from build123d import *

# Parameters (mm, degrees)
F1_DEPTH = 400
F2_R     = 2.15
F3_DEPTH = 800
F4_R     = 2


with BuildPart() as f1:
    # F0 (on Right) → F1 (new body, symmetric)
    with BuildSketch(Plane.YZ):
        Polygon((-2.5, 10), (-10, 10), (-10, 2.5), (-3.65, 2.5), (-3.65, -2.5), (-10, -2.5), (-10, -10), (-2.5, -10), (-2.5, -3.65), (2.5, -3.65), (2.5, -10), (10, -10), (10, -2.5), (3.65, -2.5), (3.65, 2.5), (10, 2.5), (10, 10), (2.5, 10), (2.5, 3.65), (-2.5, 3.65), align=None)
    extrude(amount=F1_DEPTH, both=True)

    # F2 (on face) → F3 (cut)
    with BuildSketch(Plane(origin=(-400, 0, 0), x_dir=(0, -1, 0), z_dir=(-1, 0, 0))):
        Circle(F2_R)
    extrude(amount=-F3_DEPTH, mode=Mode.SUBTRACT)

    # F4
    f4_edges = [f1.edges().sort_by_distance(p)[0] for p in [
        (0, 10, -10),
        (0, -10, -10),
        (0, -10, 10),
        (0, 10, 10),
    ]]
    fillet(f4_edges, radius=F4_R)


solid = f1.part
The listing builds one solid part. Answer for the finished solid, in the listing's coordinates (mm). Give positions to 0.01 mm unless a question says otherwise; leave off trailing zeros. Loops run counter-clockwise (first coordinate to the right, second up) from the corner with the lowest first, then second, coordinate; pieces in that order, holes last. Notation, with made-up numbers: M 53,83.25 L 87,83.25 A27 ccw 87,101.25 Z; hole C 87,45.5 d8. An arc over 180 degrees is marked long. Answer as CSV lines item,"result".
Item 1: Given pin 1 Ø1.5 at (x, y) = (-124.5, 0) entering from +Z; pin 2 Ø5.5 at (x, z) = (127, 0.5) entering from +Y; pin 3 Ø1.5 at (x, z) = (173.5, -0.5) entering from -Y; pin 4 Ø2.5 at (x, y) = (-121, -1) entering from -Z, each flat-ended and moving along its own axis, determine where each tip first touches the part or whether it passes through.
Values follow:
pin 1,"stops at z = 3.65"
pin 2,"stops at y = 10"
pin 3,"stops at y = -3.65"
pin 4,"stops at z = -3.65"
Item 2: Straight lines are drawn through the part: line 1 along Z through (x, y) = (108.5, 7); line 2 along Z through (x, y) = (-129.5, 0). For each, find the intervals that lie inside material, in ascending order. Write a range as [from, to].
Values follow:
line 1,"z = [-10, -2.5], [2.5, 10]"
line 2,"z = [-3.65, -2.15], [2.15, 3.65]"
Item 3: The part is cut by section A-A (x = 268). Give the vertices of the cut face in (y, z).
Values follow:
outline,"M -10,-8 A2 ccw -8,-10 L -2.5,-10 L -2.5,-3.65 L 2.5,-3.65 L 2.5,-10 L 8,-10 A2 ccw 10,-8 L 10,-2.5 L 3.65,-2.5 L 3.65,2.5 L 10,2.5 L 10,8 A2 ccw 8,10 L 2.5,10 L 2.5,3.65 L -2.5,3.65 L -2.5,10 L -8,10 A2 ccw -10,8 L -10,2.5 L -3.65,2.5 L -3.65,-2.5 L -10,-2.5 Z; hole C 0,0 d4.3"
